from build123d import *

# Parameters (mm, degrees)
SKETCH1_R             = 7.175
SKETCH1_R_2           = 4
BOSS_EXTRUDE1_DEPTH   = 2.54
BOSS_EXTRUDE2_START   = 2.54
SKETCH1_3_R           = 7.175
SKETCH1_3_R_2         = 4
BOSS_EXTRUDE2_DEPTH   = 6.35
F_8_CLEARANCE_HOLE1_D = 4.4958


with BuildPart() as part:
    # Sketch1 → Boss-Extrude1 (new body)
    # profile 1 of 7: a face of its own
    with BuildSketch(Plane(origin=(0, 0, 0), x_dir=(1, 0, 0), z_dir=(0, 1, 0))):
        with BuildLine():
            ThreePointArc((-6.35, -12.7), (-9.526522643, -7.199859868), (-15.878044557, -7.202497586))
            ThreePointArc((-15.878044557, -7.202497586), (-16.512685104, -7.734059372), (-17.190128061, -8.209871939))
            ThreePointArc((-17.190128061, -8.209871939), (-17.190128061, -17.190128061), (-8.209871939, -17.190128061))
            ThreePointArc((-8.209871939, -17.190128061), (-7.734059372, -16.512685104), (-7.202497586, -15.878044557))
            ThreePointArc((-7.202497586, -15.878044557), (-6.566826257, -14.345199026), (-6.35, -12.7))
        make_face()
    # profile 2 of 7: a face of its own
    with BuildSketch(Plane(origin=(0, 0, 0), x_dir=(1, 0, 0), z_dir=(0, 1, 0))):
        with BuildLine():
            ThreePointArc((7.202497586, 15.878044557), (0, 12.7), (-7.202497586, 15.878044557))
            ThreePointArc((-7.202497586, 15.878044557), (-6.566826257, 14.345199026), (-6.35, 12.7))
            ThreePointArc((-6.35, 12.7), (-9.526522643, 7.199859868), (-15.878044557, 7.202497586))
            ThreePointArc((-15.878044557, 7.202497586), (-12.7, 0), (-15.878044557, -7.202497586))
            ThreePointArc((-15.878044557, -7.202497586), (-9.526522643, -7.199859868), (-6.35, -12.7))
            ThreePointArc((-6.35, -12.7), (-6.566826257, -14.345199026), (-7.202497586, -15.878044557))
            ThreePointArc((-7.202497586, -15.878044557), (0, -12.7), (7.202497586, -15.878044557))
            ThreePointArc((7.202497586, -15.878044557), (8.209871939, -8.209871939), (15.878044557, -7.202497586))
            ThreePointArc((15.878044557, -7.202497586), (12.7, 0), (15.878044557, 7.202497586))
            ThreePointArc((15.878044557, 7.202497586), (8.209871939, 8.209871939), (7.202497586, 15.878044557))
        make_face()
        Circle(SKETCH1_R, mode=Mode.SUBTRACT)
    # profile 3 of 7: a face of its own
    with BuildSketch(Plane(origin=(0, 0, 0), x_dir=(1, 0, 0), z_dir=(0, 1, 0))):
        with BuildLine():
            ThreePointArc((17.190128061, -8.209871939), (16.512685104, -7.734059372), (15.878044557, -7.202497586))
            ThreePointArc((15.878044557, -7.202497586), (8.209871939, -8.209871939), (7.202497586, -15.878044557))
            ThreePointArc((7.202497586, -15.878044557), (7.734059372, -16.512685104), (8.209871939, -17.190128061))
            ThreePointArc((8.209871939, -17.190128061), (15.130039796, -18.566635031), (19.05, -12.7))
            ThreePointArc((19.05, -12.7), (18.566635031, -10.269960204), (17.190128061, -8.209871939))
        make_face()
    # profile 4 of 7: a face of its own
    with BuildSketch(Plane(origin=(0, 0, 0), x_dir=(1, 0, 0), z_dir=(0, 1, 0))):
        with BuildLine():
            ThreePointArc((8.209871939, 17.190128061), (7.734059372, 16.512685104), (7.202497586, 15.878044557))
            ThreePointArc((7.202497586, 15.878044557), (8.209871939, 8.209871939), (15.878044557, 7.202497586))
            ThreePointArc((15.878044557, 7.202497586), (16.512685104, 7.734059372), (17.190128061, 8.209871939))
            ThreePointArc((17.190128061, 8.209871939), (18.566635031, 10.269960204), (19.05, 12.7))
            ThreePointArc((19.05, 12.7), (15.130039796, 18.566635031), (8.209871939, 17.190128061))
        make_face()
    # profile 5 of 7: a face of its own
    with BuildSketch(Plane(origin=(0, 0, 0), x_dir=(1, 0, 0), z_dir=(0, 1, 0))):
        Circle(SKETCH1_R)
        Circle(SKETCH1_R_2, mode=Mode.SUBTRACT)
    # profile 6 of 7: a face of its own
    with BuildSketch(Plane(origin=(0, 0, 0), x_dir=(1, 0, 0), z_dir=(0, 1, 0))):
        Circle(SKETCH1_R_2)
    # profile 7 of 7: a face of its own
    with BuildSketch(Plane(origin=(0, 0, 0), x_dir=(1, 0, 0), z_dir=(0, 1, 0))):
        with BuildLine():
            ThreePointArc((-7.202497586, 15.878044557), (-7.734059372, 16.512685104), (-8.209871939, 17.190128061))
            ThreePointArc((-8.209871939, 17.190128061), (-17.190128061, 17.190128061), (-17.190128061, 8.209871939))
            ThreePointArc((-17.190128061, 8.209871939), (-16.512685104, 7.734059372), (-15.878044557, 7.202497586))
            ThreePointArc((-15.878044557, 7.202497586), (-9.526522643, 7.199859868), (-6.35, 12.7))
            ThreePointArc((-6.35, 12.7), (-6.566826257, 14.345199026), (-7.202497586, 15.878044557))
        make_face()
    extrude(amount=BOSS_EXTRUDE1_DEPTH)

    # Sketch1<3> → Boss-Extrude2 (add)
    with BuildSketch(Plane(origin=(0, 0, 0), x_dir=(1, 0, 0), z_dir=(0, 1, 0)).offset(BOSS_EXTRUDE2_START)):
        with Locations(Location((0, 0, 0), (0, 0, 270))):
            Circle(SKETCH1_3_R)
        with Locations(Location((0, 0, 0), (0, 0, 270))):
            Circle(SKETCH1_3_R_2, mode=Mode.SUBTRACT)
    extrude(amount=BOSS_EXTRUDE2_DEPTH)

    # #8 Clearance Hole1 (through all)
    with Locations(Plane(origin=(0, 2.54, 0), x_dir=(1, 0, 0), z_dir=(0, 1, 0))):
        with Locations((-12.7, 12.7), (12.7, 12.7), (12.7, -12.7), (-12.7, -12.7)):
            Hole(F_8_CLEARANCE_HOLE1_D / 2)


solid = part.part
Source: CAD feature listing. Evaluate the final solid. Frame: model axes, mm. A direction names the side the tool comes from. Coordinates: 2 decimals unless noted, no trailing zeros. Loops run counter-clockwise (first coordinate to the right, second up) from the corner with the lowest first, then second, coordinate; pieces in that order, holes last. Notation, with made-up numbers: (74, -38) - (92, -38) arc R16 ccw to (92, -21) - close; hole circle Ø2 at (42.5, 43.5). An arc over 180 degrees is marked (long way). Return JSON: item names as keys, results as strings.
Q1. Section B-B, the plane x = 0. Return loops of the section in (y, z) (3 decimals).
Results:
{"outline": "(0, -12.7) - (2.54, -12.7) - (2.54, -7.175) - (8.89, -7.175) - (8.89, -4) - (2.54, -4) - (2.54, 4) - (8.89, 4) - (8.89, 7.175) - (2.54, 7.175) - (2.54, 12.7) - (0, 12.7) - close"}
Q2. Section D-D, the plane z = -11.5. Return loops of the section in (x, y), plus the area to 3 significant figures.
Results:
{"outline": "(-18.94, 0) - (-14.6, 0) - (-14.6, 2.54) - (-18.94, 2.54) - close; (-10.8, 0) - (10.8, 0) - (10.8, 2.54) - (-10.8, 2.54) - close; (14.6, 0) - (18.94, 0) - (18.94, 2.54) - (14.6, 2.54) - close", "area": "76.9 mm2"}
Q3. Mould query, pull axis Z, two halves, no side actions, for faces 3 (the flat face through (8, 2.54, 0)), 4 (the cylindrical face through (-10.92, 1.25, 14.07)), 5 (the cylindrical face through (6.05, 5.67, 3.86)), 6 (the cylindrical face through (13.187, 1.252, 14.894)). Classes: released by +Z, released by -Z, zero draft, split by the parting line, or undercut.
Results:
{"face 3": "zero draft", "face 4": "undercut", "face 5": "split by the parting line", "face 6": "undercut"}
Q4. Access query for faces 1 (the cylindrical face through (-3.905, 5.671, -0.867)), 2 (the cylindrical face through (-17.09, 1.25, -17.29)). Directions: +Z, -Z, +X, -X, +Y, -Y. A direction counts if a zero-diameter tool reaches every point of the face in a straight line with its end or side. Return the directions, or none.
Results:
{"face 1": "+Y", "face 2": "+Y, -Y"}
Q5. Section A-A, the plane z = 0. Return loops of the section in (x, y) (3 decimals), plus the area to 3 significant figures.
Results:
{"outline": "(-12.7, 0) - (12.7, 0) - (12.7, 2.54) - (7.175, 2.54) - (7.175, 8.89) - (4, 8.89) - (4, 2.54) - (-4, 2.54) - (-4, 8.89) - (-7.175, 8.89) - (-7.175, 2.54) - (-12.7, 2.54) - close", "area": "105 mm2"}
Q6. Contact query for flat-ended pins moving along their axis: P1, Ø6.5, axis at x = 0, z = 0, coming from the +Y side; P2, Ø2, axis at x = -9, y = 7, coming from the +Z side; P3, Ø4, axis at x = -3, y = 6.5, coming from the +Z side (3 decimals); P4, Ø4, axis at y = 5, z = -6, coming from the -X side. Output: stop coordinate, or through.
Results:
{"P1": "y = 2.54", "P2": "through", "P3": "z = 7.105", "P4": "x = -5.96"}
Q7. Material intervals for line 1 along X through (y, z) = (5.5, 0) (3 decimals); line 2 along X through (y, z) = (2.5, -11.5); line 3 along Y through (x, z) = (7.5, 11.5), sorted ascending.
Results:
{"line 1": "-7.175 to -4, 4 to 7.175", "line 2": "-18.94 to -14.6, -10.8 to 10.8, 14.6 to 18.94", "line 3": "0 to 2.54"}
Q8. Section C-C, the plane y = 3.5. Return loops of the section in (x, z) (3 decimals).
Results:
{"outline": "circle Ø14.35 at (0, 0); hole circle Ø8 at (0, 0)"}
